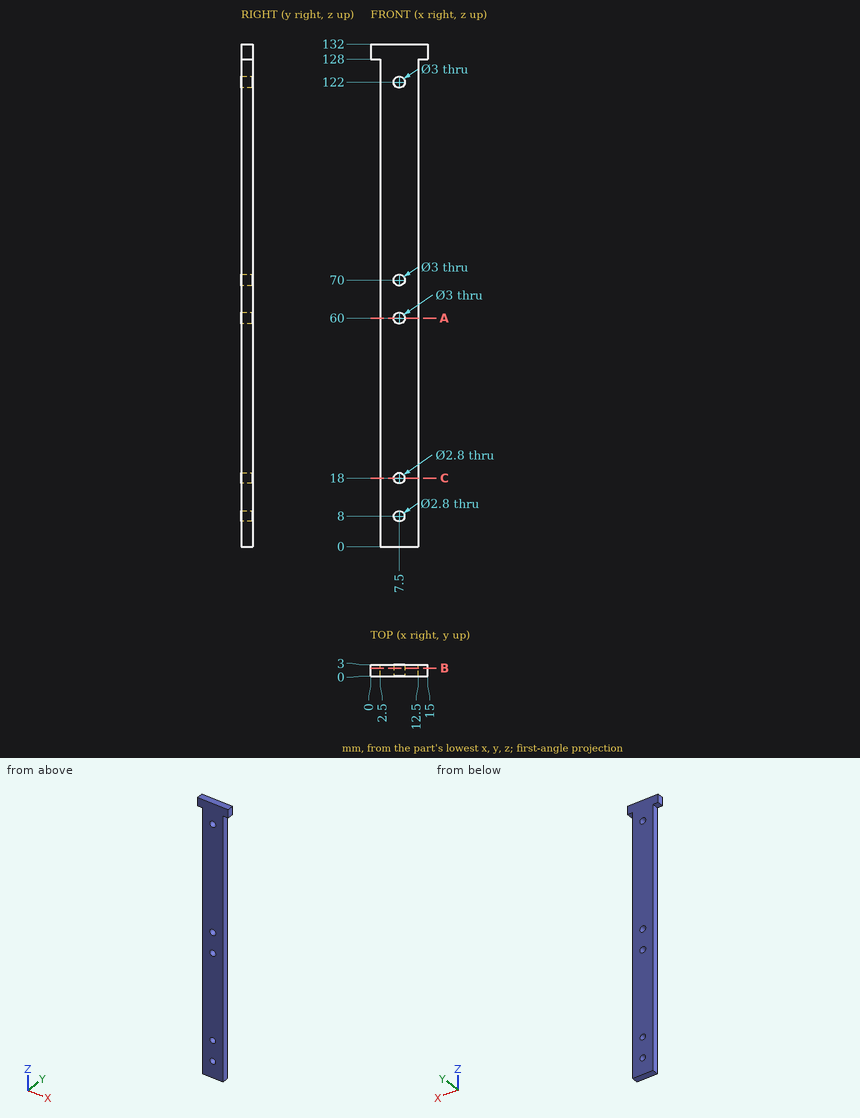
Print and shaded views of the part. All mm, measured from the part's lowest x, y and z. Coordinates: 2 decimals unless noted, no trailing zeros. Loops run counter-clockwise (first coordinate to the right, second up) from the corner with the lowest first, then second, coordinate; pieces in that order, holes last. Notation, with made-up numbers: (69.5, 37.5) -> (125.5, 37.5) arc R21 ccw to (125.5, 42.5) -> close; hole circle Ø8 at (47, 4). An arc over 180 degrees is marked (long way). Use one line per item in the form item = value. Start each with the question number.
(1) Cut at A-A on z = 60. Give the cut face in (x, y), and give its area (3 significant figures).
(2) Cut at C-C on z = 18. Give the cut face in (x, y).
(3) Flat gauge pins, fed straight in: pin 1 (6 mm diameter, centred on x = 5.5, z = 60.5, fed in from -Y); pin 2 (0.9 mm diameter, centred on y = 1, z = 61.5, fed in from -X). Where does each tip first touch, or does it go through?
(4) Cut at B-B on y = 2.05. Give the cut face in (x, z), and give its area (3 significant figures).
(5) Probe probe 1 along Z at (x, y) = (8.25, 2.8); probe 2 along X at (y, z) = (1.85, 8); probe 3 along X at (y, z) = (2.3, 60). List the from-to ranges inside material, lowest first. Write a range as from..to.
Values:
q1.outline = (2.5, 0) -> (6, 0) -> (6, 3) -> (2.5, 3) -> close; (9, 0) -> (12.5, 0) -> (12.5, 3) -> (9, 3) -> close
q1.area = 21.0 mm2
q2.outline = (2.5, 0) -> (6.1, 0) -> (6.1, 3) -> (2.5, 3) -> close; (8.9, 0) -> (12.5, 0) -> (12.5, 3) -> (8.9, 3) -> close
q3.pin_1 = 0
q3.pin_2 = 2.5
q4.outline = (0, 128) -> (2.5, 128) -> (2.5, 0) -> (12.5, 0) -> (12.5, 128) -> (15, 128) -> (15, 132) -> (0, 132) -> close; hole circle Ø3 at (7.5, 60); hole circle Ø3 at (7.5, 70); hole circle Ø3 at (7.5, 122); hole circle Ø2.8 at (7.5, 8); hole circle Ø2.8 at (7.5, 18)
q4.area = 1,310 mm2
q5.probe_1 = 0..6.82, 9.18..16.82, 19.18..58.7, 61.3..68.7, 71.3..120.7, 123.3..132
q5.probe_2 = 2.5..6.1, 8.9..12.5
q5.probe_3 = 2.5..6, 9..12.5
